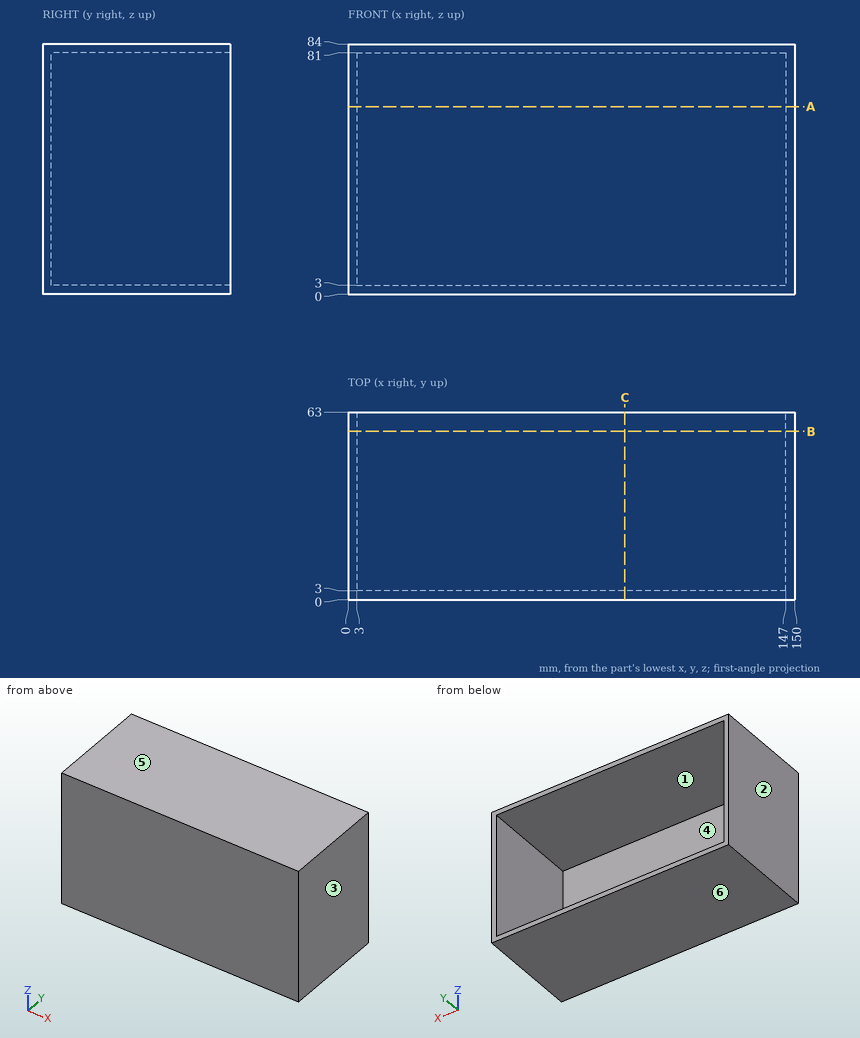
Geometry check sheet. Reference: drawing and pictorial views, mm from the part's lowest x, y, z. A direction names the side the tool comes from. Give positions to 0.01 mm unless a question says otherwise; leave off trailing zeros. Write each loop counter-clockwise with the first axis right and the second up, starting at its lowest first coordinate (ties: lowest second). Pieces come first, ordered by that corner, then holes. Notation, with made-up numbers: (81.25, 60.25) -> (103.25, 60.25) arc R11 cw to (103.25, 74.25) -> close; hole circle Ø1 at (41, 32). An arc over 180 degrees is marked (long way). One line per item, written item: value. Start each with the question number.
Item 1: Gauge pin test, flat end, axial feed: pin 1 (8 mm diameter, centred on x = 88, z = 37.5, fed in from +Y). Record the tip position at first contact, or that the pin passes through.
Item 2: Material ranges on probe 1 along X at (y, z) = (26, 23); probe 2 along Z at (x, y) = (30, 31); probe 3 along Y at (x, z) = (59.5, 47), recorded low to high. Write a range as from..to.
Item 3: Section check B-B on y = 56.5. Record the cut outline in (x, z).
Item 4: Draft check along Z on the marked faces 3, 4, 5 and 6. Enter one of: +Z half, -Z half, draft (parallel to the pull), parting line (faces both ways), or undercut.
Item 5: Tool access check on the marked faces 1 and 2. Record the directions out of +Z, -Z, +X, -X, +Y, -Y that give a thin tool (end or side, any length) a straight path to the whole face; none if there is none.
Item 6: Section check C-C on x = 93. Record the cut outline in (y, z).
Item 7: Section check A-A on z = 63. Record the cut outline in (x, y), then the cut area to 3 significant figures.
Results list:
1. pin 1: y = 3
2. probe 1: 0..3, 147..150
2. probe 2: 0..3, 81..84
2. probe 3: 0..3
3. outline: (0, 0) -> (150, 0) -> (150, 84) -> (0, 84) -> close; hole (3, 3) -> (147, 3) -> (147, 81) -> (3, 81) -> close
4. face 3: draft
4. face 4: undercut
4. face 5: +Z half
4. face 6: -Z half
5. face 1: +Y
5. face 2: +Z, -Z, -X, +Y, -Y
6. outline: (0, 0) -> (63, 0) -> (63, 3) -> (3, 3) -> (3, 81) -> (63, 81) -> (63, 84) -> (0, 84) -> close
7. outline: (0, 0) -> (150, 0) -> (150, 63) -> (147, 63) -> (147, 3) -> (3, 3) -> (3, 63) -> (0, 63) -> close
7. area: 810 mm²
